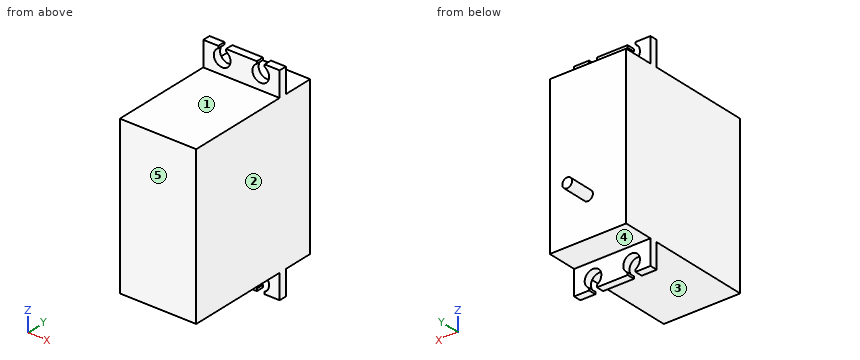
from build123d import *

# Parameters (mm, degrees)
SKETCH1_W           = 19.8
SKETCH1_H           = 40.6
BOSS_EXTRUDE1_DEPTH = 36.6
SKETCH2_R           = 1.27
BOSS_EXTRUDE2_DEPTH = 6.700000022
SKETCH3_W           = 19.8
SKETCH3_H           = 2
BOSS_EXTRUDE3_DEPTH = 6.4
SKETCH4_W           = 19.8
SKETCH4_H           = 2
BOSS_EXTRUDE4_DEPTH = 6.4
CUT_EXTRUDE1_DEPTH  = 47.37305252


with BuildPart() as part:
    # Sketch1 → Boss-Extrude1 (new body)
    with BuildSketch(Plane(origin=(0, 0, 0), x_dir=(1, 0, 0), z_dir=(0, 1, 0))):
        Rectangle(SKETCH1_W, SKETCH1_H)
    extrude(amount=BOSS_EXTRUDE1_DEPTH)

    # Sketch2 → Boss-Extrude2 (add)
    with BuildSketch(Plane(origin=(0, 36.6, 0), x_dir=(1, 0, 0), z_dir=(0, 1, 0))):
        with Locations(Location((0, 10.3, 0), (0, 0, 90))):
            Circle(SKETCH2_R)
    extrude(amount=BOSS_EXTRUDE2_DEPTH)

    # Sketch3 → Boss-Extrude3 (add)
    with BuildSketch(Plane(origin=(0, 0, -20.3), x_dir=(-1, 0, 0), z_dir=(0, 0, -1))):
        with Locations((0, 27.8)):
            Rectangle(SKETCH3_W, SKETCH3_H)
    extrude(amount=BOSS_EXTRUDE3_DEPTH)

    # Sketch4 → Boss-Extrude4 (add)
    with BuildSketch(Plane.XY.offset(20.3)):
        with Locations((0, 27.8)):
            Rectangle(SKETCH4_W, SKETCH4_H)
    extrude(amount=BOSS_EXTRUDE4_DEPTH)

    # Sketch5 → Cut-Extrude1 (cut, through all)
    with BuildSketch(Plane(origin=(0, 36.6, 0), x_dir=(1, 0, 0), z_dir=(0, 1, 0))):
        with BuildLine():
            Line((-6.016, 26.105), (-6.016, 26.7))
            Line((-6.016, 26.7), (-3.984, 26.7))
            Line((-3.984, 26.7), (-3.984, 26.105))
            ThreePointArc((-3.984, 26.105), (-5, 22.041), (-6.016, 26.105))
        make_face()
        with BuildLine():
            Line((3.984, 26.105), (3.984, 26.7))
            Line((3.984, 26.7), (6.016, 26.7))
            Line((6.016, 26.7), (6.016, 26.105))
            ThreePointArc((6.016, 26.105), (5, 22.041), (3.984, 26.105))
        make_face()
        with BuildLine():
            Line((-6.016, -26.105), (-6.016, -26.7))
            Line((-6.016, -26.7), (-3.984, -26.7))
            Line((-3.984, -26.7), (-3.984, -26.105))
            ThreePointArc((-3.984, -26.105), (-5, -22.041), (-6.016, -26.105))
        make_face()
        with BuildLine():
            Line((3.984, -26.105), (3.984, -26.7))
            Line((3.984, -26.7), (6.016, -26.7))
            Line((6.016, -26.7), (6.016, -26.105))
            ThreePointArc((6.016, -26.105), (5, -22.041), (3.984, -26.105))
        make_face()
    extrude(amount=-CUT_EXTRUDE1_DEPTH, mode=Mode.SUBTRACT)


solid = part.part
Part model, mm, in its own coordinate system. Face numbers are marked on the shaded views. A direction names the side the tool comes from. Coordinates: 2 decimals unless noted, no trailing zeros. Order: outer loops, then holes, each group sorted by start corner. A loop starts at its lowest first (then second) coordinate and runs counter-clockwise, first axis right, second up.
(1) Slice it at D-D, the plane z = -10.3. Write the cut outline in (x, y).
Check sheet entries:
outline: (-9.9, 0) - (9.9, 0) - (9.9, 36.6) - (1.27, 36.6) - (1.27, 43.3) - (-1.27, 43.3) - (-1.27, 36.6) - (-9.9, 36.6) - close
(2) Pin check, flat tips, straight feed: pin 1 Ø3 at (x, z) = (0, -22.5) entering from -Y; pin 2 Ø3 at (x, z) = (1.5, -22.5) entering from +Y; pin 3 Ø4 at (x, y) = (1, 14.5) entering from +Z. Stop position of each tip, or through.
Check sheet entries:
pin 1: stops at y = 26.8
pin 2: stops at y = 28.8
pin 3: stops at z = 20.3
(3) Slice it at A-A, the plane z = -24.2. Write the cut outline in (x, y), and give its area (3 significant figures).
Check sheet entries:
outline: (-9.9, 26.8) - (-7.16, 26.8) - (-7.16, 28.8) - (-9.9, 28.8) - close; (-2.84, 26.8) - (2.84, 26.8) - (2.84, 28.8) - (-2.84, 28.8) - close; (7.16, 26.8) - (9.9, 26.8) - (9.9, 28.8) - (7.16, 28.8) - close
area: 22.3 mm2
(4) Probe L1, parallel to X at y = 27.3, z = 24.2; L2, parallel to X at y = 28, z = -24; L3, parallel to Y at x = -8, z = -5.5. List the from-to ranges inside material, lowest first.
Check sheet entries:
L1: x = -9.9 to -7.16, -2.84 to 2.84, 7.16 to 9.9
L2: x = -9.9 to -7.15, -2.85 to 2.85, 7.15 to 9.9
L3: y = 0 to 36.6
(5) Slice it at C-C, the plane y = 39.5. Write the cut outline in (x, z), and give its area (3 significant figures).
Check sheet entries:
outline: circle Ø2.54 at (0, -10.3)
area: 5.07 mm2
(6) Tool access for the marked faces 1, 2, 3, 4 and 5: list every direction of +Z, -Z, +X, -X, +Y, -Y with a clear straight run to the whole face (end or side of a thin tool).
Check sheet entries:
face 1: +Z, +X, -X, -Y
face 2: +Z, -Z, +X, +Y, -Y
face 3: -Z, +X, -X, -Y
face 4: -Z, +X, -X, +Y
face 5: +Z, -Z, +X, -X, -Y
(7) Slice it at B-B, the plane x = 0. Write the cut outline in (y, z).
Check sheet entries:
outline: (0, -20.3) - (26.8, -20.3) - (26.8, -26.7) - (28.8, -26.7) - (28.8, -20.3) - (36.6, -20.3) - (36.6, -11.57) - (43.3, -11.57) - (43.3, -9.03) - (36.6, -9.03) - (36.6, 20.3) - (28.8, 20.3) - (28.8, 26.7) - (26.8, 26.7) - (26.8, 20.3) - (0, 20.3) - close
